Print and shaded views of the part. All mm, measured from the part's lowest x, y and z. A direction names the side the tool comes from. Round coordinates to 2 decimals unless told otherwise and drop trailing zeros. Loops run counter-clockwise (first coordinate to the right, second up) from the corner with the lowest first, then second, coordinate; pieces in that order, holes last. Notation, with made-up numbers: (-1, 48.25) -> (24, 48.25) arc R16 cw to (24, 52.25) -> close; hole circle Ø7 at (-35.5, 28). An arc over 180 degrees is marked (long way). Use a Markdown table: item, result.
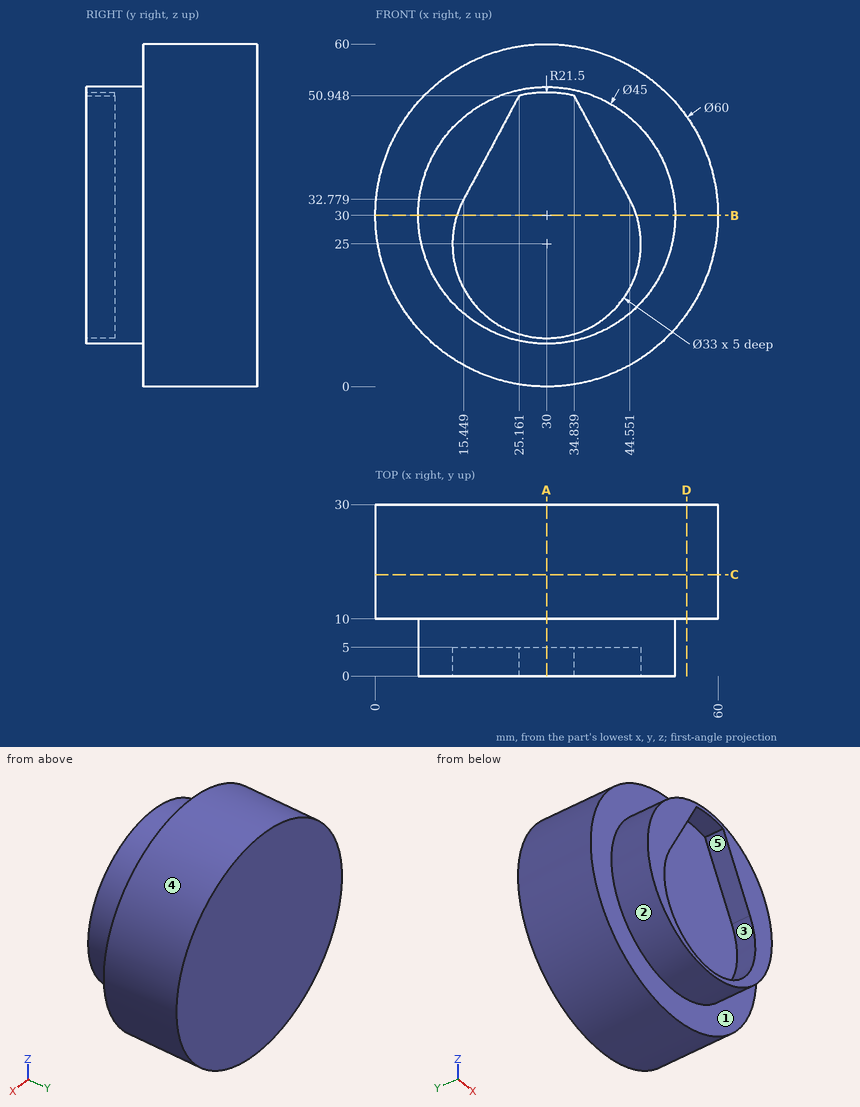
Q1. Flat gauge pins, fed straight in: pin 1 (10 mm diameter, centred on x = 52, y = 26.5, fed in from -Z); pin 2 (10 mm diameter, centred on x = 16, y = 26.5, fed in from +Z); pin 3 (4 mm diameter, centred on x = 22, y = 19, fed in from -Z). Where does each tip first touch, or does it go through?
Results list:
| item | result |
|---|---|
| pin 1 | stops at z = 5.28 |
| pin 2 | stops at z = 58.62 |
| pin 3 | stops at z = 0.61 |
Q2. Drill centre lines: L1, parallel to Y at x = 30, z = 38.5; L2, parallel to X at y = 3.5, z = 40 (1 decimal); L3, parallel to Y at x = 34.5, z = 5.5. Where is each one in solid material? Low to high. Write a range as from..to.
Results list:
| item | result |
|---|---|
| L1 | y = 5..30 |
| L2 | x = 9.8..19.3, 40.7..50.2 |
| L3 | y = 10..30 |
Q3. Tool access for the marked faces 4 and 5: list every direction of +Z, -Z, +X, -X, +Y, -Y with a clear straight run to the whole face (end or side of a thin tool).
Results list:
| item | result |
|---|---|
| face 4 | +Y, -Y |
| face 5 | -Y |
Q4. Pull direction X, two halves, no side cores. Call the marked faces 1, 2 and 3: released by +X, released by -X, zero draft, split by the parting line, or undercut.
Results list:
| item | result |
|---|---|
| face 1 | zero draft |
| face 2 | split by the parting line |
| face 3 | undercut |
Q5. Band-saw the part on D-D, the plane x = 54.5. Give the cut face in (y, z).
Results list:
| item | result |
|---|---|
| outline | (10, 12.69) -> (30, 12.69) -> (30, 47.31) -> (10, 47.31) -> close |
Q6. Band-saw the part on B-B, the plane z = 30. Give the cut face in (x, y) (1 decimal).
Results list:
| item | result |
|---|---|
| outline | (0, 10) -> (7.5, 10) -> (7.5, 0) -> (14.3, 0) -> (14.3, 5) -> (45.7, 5) -> (45.7, 0) -> (52.5, 0) -> (52.5, 10) -> (60, 10) -> (60, 30) -> (0, 30) -> close |
Q7. Band-saw the part on C-C, the plane y = 17.75. Give the cut face in (x, z).
Results list:
| item | result |
|---|---|
| outline | circle Ø60 at (30, 30) |
Q8. Band-saw the part on A-A, the plane x = 30. Give the cut face in (y, z), plus the area to 4 significant figures.
Results list:
| item | result |
|---|---|
| outline | (0, 7.5) -> (10, 7.5) -> (10, 0) -> (30, 0) -> (30, 60) -> (10, 60) -> (10, 52.5) -> (0, 52.5) -> (0, 51.5) -> (5, 51.5) -> (5, 8.5) -> (0, 8.5) -> close |
| area | 1,435 mm² |
